Read the model definition and answer for the solid it produces. Units are mm, in the model's axes. A direction names the side the tool comes from. Coordinates: 2 decimals unless noted, no trailing zeros. Loops run counter-clockwise (first coordinate to the right, second up) from the corner with the lowest first, then second, coordinate; pieces in that order, holes last. Notation, with made-up numbers: (2, 88.25) -> (59, 88.25) arc R28 cw to (59, 124.25) -> close; hole circle Ø1 at (2, -18). An arc over 180 degrees is marked (long way). Answer as CSV lines item,"result".
```python
from build123d import *

# Parameters (mm, degrees)
F0_R     = 1.6
F1_DEPTH = 1.5


with BuildPart() as f1:
    # F0 (on Front) → F1 (new body)
    with BuildSketch(Plane.XZ):
        with BuildLine():
            Line((25.154329, 22.928932), (16.970563, 31.112698))
            Line((16.970563, 31.112698), (13.300916, 27.844789))
            ThreePointArc((13.300916, 27.844789), (0, 22.78084), (-13.300916, 27.844789))
            Line((-13.300916, 27.844789), (-16.970563, 31.112698))
            Line((-16.970563, 31.112698), (-27.154329, 20.928932))
            ThreePointArc((-27.154329, 20.928932), (-30.398562, 18.761205), (-34.225397, 18))
            Line((-34.225397, 18), (-36.4, 18))
            ThreePointArc((-36.4, 18), (-39.228427, 16.828427), (-40.4, 14))
            Line((-40.4, 14), (-40.4, 0))
            Line((-40.4, 0), (-40.4, -14))
            ThreePointArc((-40.4, -14), (-39.228427, -16.828427), (-36.4, -18))
            Line((-36.4, -18), (-34.225397, -18))
            ThreePointArc((-34.225397, -18), (-30.398562, -18.761205), (-27.154329, -20.928932))
            Line((-27.154329, -20.928932), (-16.970563, -31.112698))
            Line((-16.970563, -31.112698), (-13.300916, -27.844789))
            ThreePointArc((-13.300916, -27.844789), (0, -22.78084), (13.300916, -27.844789))
            Line((13.300916, -27.844789), (16.970563, -31.112698))
            Line((16.970563, -31.112698), (25.154329, -22.928932))
            ThreePointArc((25.154329, -22.928932), (28.398562, -20.761205), (32.225397, -20))
            Line((32.225397, -20), (40, -20))
            ThreePointArc((40, -20), (50.606602, -15.606602), (55, -5))
            Line((55, -5), (55, 0))
            Line((55, 0), (55, 5))
            ThreePointArc((55, 5), (50.606602, 15.606602), (40, 20))
            Line((40, 20), (32.225397, 20))
            ThreePointArc((32.225397, 20), (28.398562, 20.761205), (25.154329, 22.928932))
        make_face()
        with Locations((-13.966, -22.524)):
            Circle(F0_R, mode=Mode.SUBTRACT)
        with Locations((-7.249, -15.807)):
            Circle(F0_R, mode=Mode.SUBTRACT)
        with Locations((7.249, -15.807)):
            Circle(F0_R, mode=Mode.SUBTRACT)
        with BuildLine():
            ThreePointArc((-34.7, -9.6), (-33.65, -10.65), (-34.7, -11.7))
            Line((-34.7, -11.7), (-36.3, -11.7))
            ThreePointArc((-36.3, -11.7), (-37.35, -10.65), (-36.3, -9.6))
            Line((-36.3, -9.6), (-36.3, -7.8))
            ThreePointArc((-36.3, -7.8), (-37.35, -6.75), (-36.3, -5.7))
            Line((-36.3, -5.7), (-34.7, -5.7))
            ThreePointArc((-34.7, -5.7), (-33.65, -6.75), (-34.7, -7.8))
            Line((-34.7, -7.8), (-34.7, -9.6))
        make_face(mode=Mode.SUBTRACT)
        with Locations((-22.452, -14)):
            Circle(F0_R, mode=Mode.SUBTRACT)
        with Locations((-28.7, -5.7)):
            Circle(F0_R, mode=Mode.SUBTRACT)
        with Locations((-15.25, -15.25)):
            Circle(F0_R, mode=Mode.SUBTRACT)
        with Locations((-15.734, -7.322)):
            Circle(F0_R, mode=Mode.SUBTRACT)
        with Locations((13.966, -22.524)):
            Circle(F0_R, mode=Mode.SUBTRACT)
        with Locations((15.25, -15.25)):
            Circle(F0_R, mode=Mode.SUBTRACT)
        with Locations((22.452, -14)):
            Circle(F0_R, mode=Mode.SUBTRACT)
        with BuildLine():
            Line((30, -13.9), (32, -13.9))
            ThreePointArc((32, -13.9), (32.8, -14.7), (32, -15.5))
            Line((32, -15.5), (30, -15.5))
            ThreePointArc((30, -15.5), (29.2, -14.7), (30, -13.9))
        make_face(mode=Mode.SUBTRACT)
        with Locations((15.734, -7.322)):
            Circle(F0_R, mode=Mode.SUBTRACT)
        with Locations((42, -14)):
            Circle(F0_R, mode=Mode.SUBTRACT)
        with Locations((-28.7, 5.7)):
            Circle(F0_R, mode=Mode.SUBTRACT)
        with BuildLine():
            ThreePointArc((-34.7, 7.8), (-33.65, 6.75), (-34.7, 5.7))
            Line((-34.7, 5.7), (-36.3, 5.7))
            ThreePointArc((-36.3, 5.7), (-37.35, 6.75), (-36.3, 7.8))
            Line((-36.3, 7.8), (-36.3, 9.6))
            ThreePointArc((-36.3, 9.6), (-37.35, 10.65), (-36.3, 11.7))
            Line((-36.3, 11.7), (-34.7, 11.7))
            ThreePointArc((-34.7, 11.7), (-33.65, 10.65), (-34.7, 9.6))
            Line((-34.7, 9.6), (-34.7, 7.8))
        make_face(mode=Mode.SUBTRACT)
        with Locations((-22.452, 14)):
            Circle(F0_R, mode=Mode.SUBTRACT)
        with Locations((-15.734, 7.322)):
            Circle(F0_R, mode=Mode.SUBTRACT)
        with Locations((-15.25, 15.25)):
            Circle(F0_R, mode=Mode.SUBTRACT)
        with Locations((-7.249, 15.807)):
            Circle(F0_R, mode=Mode.SUBTRACT)
        with Locations((-13.966, 22.524)):
            Circle(F0_R, mode=Mode.SUBTRACT)
        with Locations((7.249, 15.807)):
            Circle(F0_R, mode=Mode.SUBTRACT)
        with Locations((15.734, 7.322)):
            Circle(F0_R, mode=Mode.SUBTRACT)
        with Locations((15.25, 15.25)):
            Circle(F0_R, mode=Mode.SUBTRACT)
        with Locations((22.452, 14)):
            Circle(F0_R, mode=Mode.SUBTRACT)
        with BuildLine():
            ThreePointArc((30, 13.9), (29.2, 14.7), (30, 15.5))
            Line((30, 15.5), (32, 15.5))
            ThreePointArc((32, 15.5), (32.8, 14.7), (32, 13.9))
            Line((32, 13.9), (30, 13.9))
        make_face(mode=Mode.SUBTRACT)
        with BuildLine():
            Line((28, -4.5), (28, 0))
            Line((28, 0), (28, 4.5))
            ThreePointArc((28, 4.5), (29.464466, 8.035534), (33, 9.5))
            Line((33, 9.5), (42, 9.5))
            ThreePointArc((42, 9.5), (45.535534, 8.035534), (47, 4.5))
            Line((47, 4.5), (47, 0))
            Line((47, 0), (47, -4.5))
            ThreePointArc((47, -4.5), (45.535534, -8.035534), (42, -9.5))
            Line((42, -9.5), (33, -9.5))
            ThreePointArc((33, -9.5), (29.464466, -8.035534), (28, -4.5))
        make_face(mode=Mode.SUBTRACT)
        with Locations((42, 14)):
            Circle(F0_R, mode=Mode.SUBTRACT)
        with Locations((13.966, 22.524)):
            Circle(F0_R, mode=Mode.SUBTRACT)
    extrude(amount=F1_DEPTH)


solid = f1.part
```
Q1. A cutting plane is placed at C-C, the plane x = 4. Write down the section's boundary in (y, z), and give its area (3 significant figures).
Results:
outline,"(-1.5, -23.18) -> (0, -23.18) -> (0, 23.18) -> (-1.5, 23.18) -> close"
area,"69.6 mm²"
Q2. Find the intervals of material crossed by probe 1 along Z at (x, y) = (7, -1.2); probe 2 along Z at (x, y) = (-36, -0.3); probe 3 along X at (y, z) = (-0.9, 17), in increasing order. Write a range as [from, to].
Results:
probe 1,"z = [-24.05, -17.39], [-14.23, 14.23], [17.39, 24.05]"
probe 2,"z = [-18, -11.7], [-5.7, 5.7], [11.7, 18]"
probe 3,"x = [-39.05, -8.32], [-6.18, 6.18], [8.32, 49]"
Q3. A cutting plane is placed at B-B, the plane x = 46. Write down the section's boundary in (y, z).
Results:
outline,"(-1.5, -18.75) -> (0, -18.75) -> (0, -7.5) -> (-1.5, -7.5) -> close; (-1.5, 7.5) -> (0, 7.5) -> (0, 18.75) -> (-1.5, 18.75) -> close"
Q4. For a pull along X with two mould halves and no side action, classify faces 3 (the face through (-21.991, -0.74, 26.092)), 4 (the face through (7, -1.5, 0)), 5 (the face through (28.35, -0.74, -20.78)), 6 (the face through (22.244, -0.74, 15.586)) as pulls with the +X half, pulls with the -X half, needs draft (parallel to the pull), parting line crosses it, or undercut.
Results:
face 3,"pulls with the -X half"
face 4,"needs draft"
face 5,"pulls with the +X half"
face 6,"undercut"
Q5. A cutting plane is placed at D-D, the plane y = -0.85. Give the number of separate pieces and of enclosed holes in the cut face, and give its area (3 significant figures).
Results:
separate pieces,"1"
enclosed holes,"29"
area,"3,720 mm²"
Q6. Given pin 1 Ø3 at (x, z) = (15.25, -15.25) entering from +Y; pin 2 Ø10 at (x, z) = (-23, 6) entering from +Y, each flat-ended and moving along its own axis, determine where each tip first touches the part or whether it passes through.
Results:
pin 1,"passes through"
pin 2,"stops at y = 0"
Q7. For faces 1 (the face through (50.49, -0.74, -15.72)), 2 (the face through (45.57, -0.74, -8)), determine the directions among +Z, -Z, +X, -X, +Y, -Y from which every point of the face is accessible in a straight line to the end or side of a thin tool.
Results:
face 1,"-Z, +X, +Y, -Y"
face 2,"+Y, -Y"
Q8. A cutting plane is placed at A-A, the plane z = 2.5. Write down the section's boundary in (x, y).
Results:
outline,"(-40.4, -1.5) -> (28, -1.5) -> (28, 0) -> (-40.4, 0) -> close; (47, -1.5) -> (55, -1.5) -> (55, 0) -> (47, 0) -> close"
